Source: three-view drawing plus pictorial views. Frame: mm from the lowest corner of the part. A direction names the side the tool comes from. Give positions to 0.01 mm unless a question says otherwise; leave off trailing zeros. Loops run counter-clockwise (first coordinate to the right, second up) from the corner with the lowest first, then second, coordinate; pieces in that order, holes last.
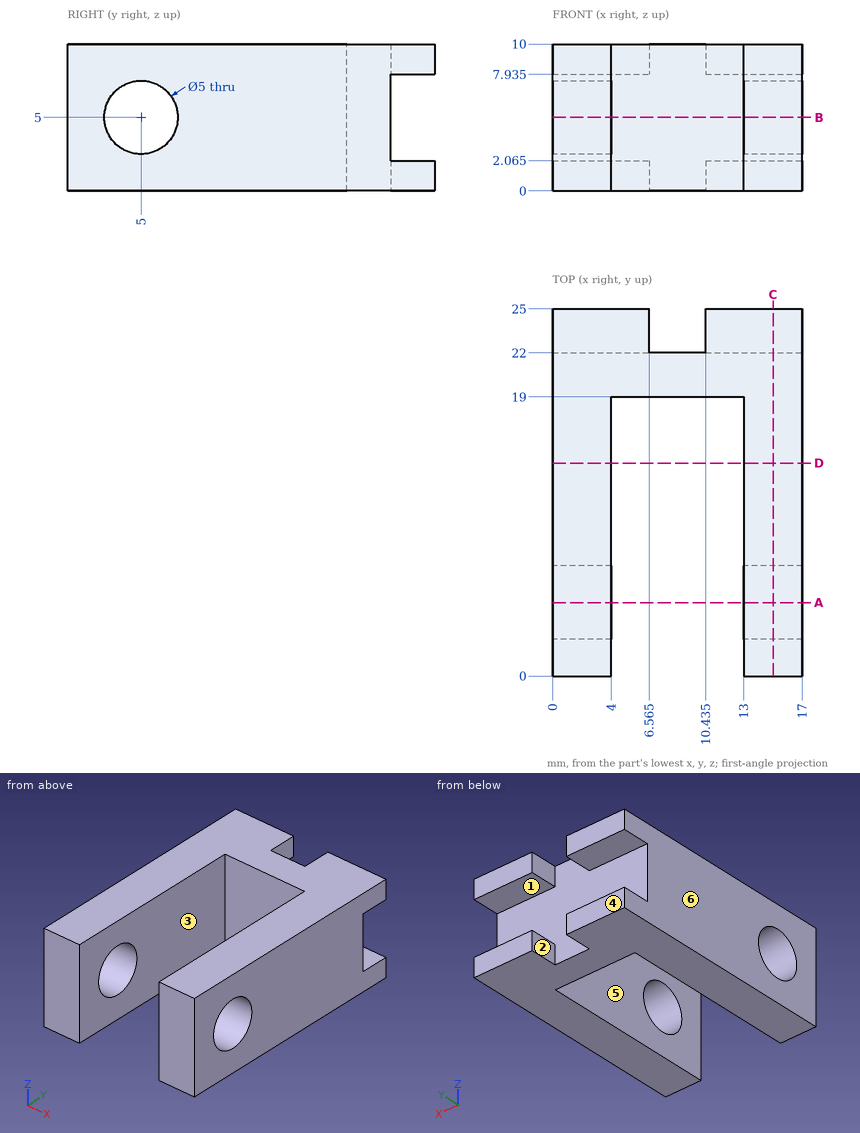
Q1. Pin query (flat end, axial travel): pin 1 Ø4 at (y, z) = (5, 5) entering from +X; pin 2 Ø3 at (x, z) = (9.5, 5) entering from +Y. Return the tip coordinate at first contact, or that it passes through.
Q2. Section query D-D, the plane y = 14.5. Return loops of the section in (x, z).
Q3. Section query B-B, the plane z = 5. Return loops of the section in (x, y).
Q4. Mould query, pull axis X, two halves, no side actions, for the marked faces 4, 5 and 6. Classes: +X half, -X half, draft (parallel to the pull), parting line (faces both ways), or undercut.
Q5. Material intervals for probe 1 along Y at (x, z) = (3.1, 5); probe 2 along X at (y, z) = (15, 8.25); probe 3 along Y at (x, z) = (5.25, 8.5), sorted ascending.
Q6. Section query A-A, the plane y = 5. Return loops of the section in (x, z), and give its area (3 significant figures).
Q7. Reachability of the marked faces 1, 2 and 3 from +Z, -Z, +X, -X, +Y, -Y: full face, straight path, thin tool, end or side. Return the list, or none.
Q8. Section query C-C, the plane x = 15. Return loops of the section in (y, z) (3 decimals), and give its area (3 significant figures).
Resolved:
1. pin 1: passes through
1. pin 2: stops at y = 22
2. outline: (0, 0) - (4, 0) - (4, 10) - (0, 10) - close; (13, 0) - (17, 0) - (17, 10) - (13, 10) - close
3. outline: (0, 0) - (4, 0) - (4, 2.5) - (0, 2.5) - close; (0, 7.5) - (4, 7.5) - (4, 19) - (13, 19) - (13, 7.5) - (17, 7.5) - (17, 22) - (0, 22) - close; (13, 0) - (17, 0) - (17, 2.5) - (13, 2.5) - close
4. face 4: draft
4. face 5: undercut
4. face 6: -X half
5. probe 1: y = 0 to 2.5, 7.5 to 22
5. probe 2: x = 0 to 4, 13 to 17
5. probe 3: y = 19 to 25
6. outline: (0, 0) - (4, 0) - (4, 2.5) - (0, 2.5) - close; (0, 7.5) - (4, 7.5) - (4, 10) - (0, 10) - close; (13, 0) - (17, 0) - (17, 2.5) - (13, 2.5) - close; (13, 7.5) - (17, 7.5) - (17, 10) - (13, 10) - close
6. area: 40.0 mm2
7. face 1: +X, -X, +Y
7. face 2: +Z, -Z, +Y
7. face 3: +Z, -Z, -Y
8. outline: (0, 0) - (25, 0) - (25, 2.065) - (22, 2.065) - (22, 7.935) - (25, 7.935) - (25, 10) - (0, 10) - close; hole circle Ø5 at (5, 5)
8. area: 213 mm2
